```python
from build123d import *

# Parameters (mm, degrees)
SKETCH1_R          = 20
SKETCH1_R_2        = 2.75
SKETCH1_R_3        = 6.25
BASE_FLANGE1_DEPTH = 4
FILLET1_R          = 10


# Sheet-metal steps are written as plain solids
with BuildPart() as part:
    # Sketch1 → Base-Flange1 (new body)
    with BuildSketch(Plane(origin=(0, 0, 0), x_dir=(1, 0, 0), z_dir=(0, 1, 0))):
        with BuildLine():
            Line((32.5, 32.5), (52.909362517, 6.118985584))
            ThreePointArc((52.909362517, 6.118985584), (55, 0), (52.909362517, -6.118985584))
            Line((52.909362517, -6.118985584), (32.5, -32.5))
            Line((32.5, -32.5), (-32.5, -32.5))
            Line((-32.5, -32.5), (-52.909362517, -6.118985584))
            ThreePointArc((-52.909362517, -6.118985584), (-55, 0), (-52.909362517, 6.118985584))
            Line((-52.909362517, 6.118985584), (-32.5, 32.5))
            Line((-32.5, 32.5), (32.5, 32.5))
        make_face()
        with Locations(Location((0, 0, 0), (0, 0, 270))):
            Circle(SKETCH1_R, mode=Mode.SUBTRACT)
        with Locations(Location((-23.57, 23.57, 0), (0, 0, 270))):
            Circle(SKETCH1_R_2, mode=Mode.SUBTRACT)
        with Locations(Location((23.57, 23.57, 0), (0, 0, 270))):
            Circle(SKETCH1_R_2, mode=Mode.SUBTRACT)
        with Locations(Location((23.57, -23.57, 0), (0, 0, 270))):
            Circle(SKETCH1_R_2, mode=Mode.SUBTRACT)
        with Locations(Location((-23.57, -23.57, 0), (0, 0, 270))):
            Circle(SKETCH1_R_2, mode=Mode.SUBTRACT)
        with Locations(Location((-45, 0, 0), (0, 0, 270))):
            Circle(SKETCH1_R_3, mode=Mode.SUBTRACT)
        with Locations(Location((45, 0, 0), (0, 0, 270))):
            Circle(SKETCH1_R_3, mode=Mode.SUBTRACT)
    extrude(amount=-BASE_FLANGE1_DEPTH)

    # Fillet1
    fillet1_edges = [part.edges().sort_by_distance(p)[0] for p in [
        (32.5, -2, -32.5),
        (32.5, -2, 32.5),
        (-32.5, -2, 32.5),
        (-32.5, -2, -32.5),
    ]]
    fillet(fillet1_edges, radius=FILLET1_R)


solid = part.part
```
Can you work these out from the model? Positions are in its coordinate system, mm. Round coordinates to 2 decimals unless told otherwise and drop trailing zeros. Loops run counter-clockwise (first coordinate to the right, second up) from the corner with the lowest first, then second, coordinate; pieces in that order, holes last. Notation, with made-up numbers: M 30,-11.75 L 87,-11.75 A25 ccw 87,22.25 Z; hole C -29,43 d9. An arc over 180 degrees is marked long. Answer in a Markdown table with one row per item.
1. If we section it at B-B, the plane y = -2.35: Please give me the cut outline in (x, z), plus the area to 3 significant figures.
Established:
| item | result |
|---|---|
| outline | M -52.91,-6.12 L -35.5,-28.62 A10 ccw -27.59,-32.5 L 27.59,-32.5 A10 ccw 35.5,-28.62 L 52.91,-6.12 A10 ccw 52.91,6.12 L 35.5,28.62 A10 ccw 27.59,32.5 L -27.59,32.5 A10 ccw -35.5,28.62 L -52.91,6.12 A10 ccw Z; hole C -45,0 d12.5; hole C -23.57,-23.57 d5.5; hole C -23.57,23.57 d5.5; hole C 0,0 d40; hole C 23.57,-23.57 d5.5; hole C 23.57,23.57 d5.5; hole C 45,0 d12.5 |
| area | 4,230 mm² |
2. Thinking about a two-plate mould opening in Z: for faces 1 (the face through (51.2, -2, -0.8)), 2 (the face through (-44.33, -1.97, -17.21)), 3 (the face through (-55, -2, 0)), which applies, pulls with the +Z half, pulls with the -Z half, needs draft (parallel to the pull), parting line crosses it, or undercut?
Established:
| item | result |
|---|---|
| face 1 | undercut |
| face 2 | pulls with the -Z half |
| face 3 | parting line crosses it |
3. If we section it at D-D, the plane z = -16.5: Please give me the cut outline in (x, y), plus the area to 3 significant figures.
Established:
| item | result |
|---|---|
| outline | M -44.88,-4 L -11.3,-4 L -11.3,0 L -44.88,0 Z; M 11.3,-4 L 44.88,-4 L 44.88,0 L 11.3,0 Z |
| area | 269 mm² |
4. Please list where these lines run through material, in increasing order: line 1 (X direction, y = -2.9, z = 3); line 2 (Z direction, x = 25, y = -2.3); line 3 (X direction, y = -3, z = -23.57). Write a range as from..to.
Established:
| item | result |
|---|---|
| line 1 | -54.54..-50.48, -39.52..-19.77, 19.77..39.52, 50.48..54.54 |
| line 2 | -32.5..-25.92, -21.22..21.22, 25.92..32.5 |
| line 3 | -39.41..-26.32, -20.82..20.82, 26.32..39.41 |
5. If we section it at A-A, the plane x = 0: Please give me the cut outline in (y, z).
Established:
| item | result |
|---|---|
| outline | M -4,-32.5 L 0,-32.5 L 0,-20 L -4,-20 Z; M -4,20 L 0,20 L 0,32.5 L -4,32.5 Z |
6. If we section it at C-C, the plane x = -23.57: Please give me the cut outline in (y, z), plus the area to 3 significant figures.
Established:
| item | result |
|---|---|
| outline | M -4,-32.5 L 0,-32.5 L 0,-26.32 L -4,-26.32 Z; M -4,-20.82 L 0,-20.82 L 0,20.82 L -4,20.82 Z; M -4,26.32 L 0,26.32 L 0,32.5 L -4,32.5 Z |
| area | 216 mm² |
